from build123d import *

# Parameters (mm, degrees)
SKETCH1_R              = 50
BOSS_EXTRUDE2_DEPTH    = 2
SPLIT1_SURFACE_1_BACK  = 156.576
SPLIT1_SURFACE_1_DEPTH = 313.152
SPLIT1_SURFACE_2_BACK  = 156.576
SPLIT1_SURFACE_2_DEPTH = 313.152
BODY_DELETE1_DEPTH     = 2
BOSS_EXTRUDE3_DEPTH    = 2
BOSS_EXTRUDE5_START    = -2
SKETCH4_W              = 2
SKETCH4_H              = 5
BOSS_EXTRUDE5_DEPTH    = 2


# Read off the part's stored shape, not the designer's step: Body-Delete1
with BuildPart() as part:
    # Sketch1 → Boss-Extrude2 (new body)
    with BuildSketch(Plane(origin=(0, 0, 0), x_dir=(1, 0, 0), z_dir=(0, 1, 0))):
        with BuildLine():
            Line((22.912878475, 50), (30, 50))
            Line((30, 50), (30, 55))
            Line((30, 55), (0, 55))
            ThreePointArc((0, 55), (-11.7260394, -53.735463151), (22.912878475, 50))
        make_face()
        with Locations(Location((0, 0, 0), (0, 0, 270))):
            Circle(SKETCH1_R, mode=Mode.SUBTRACT)
    extrude(amount=BOSS_EXTRUDE2_DEPTH)


with BuildPart() as body_2:
    # Split1: the piece behind the surface
    add(part.part)
    # Split1 surface: a surface, the sketch's curves swept straight by 313.152 mm
    with BuildLine(Plane(origin=(0, 2, 0), x_dir=(1, 0, 0), z_dir=(0, 1, 0)).offset(-SPLIT1_SURFACE_1_BACK), mode=Mode.PRIVATE) as split1_surface_1_path:
        Line((0, 50), (71.831983425, 50))
        Line((71.831983425, 50), (71.831983425, -59.181674134))
        Line((71.831983425, -59.181674134), (-65.509549092, -59.181674134))
        Line((-65.509549092, -59.181674134), (-65.509549092, 0))
        Line((-65.509549092, 0), (0, 0))
        Line((0, 0), (0, 50))
    split1_surface_1 = Shell.extrude(split1_surface_1_path.wire(), (0 * SPLIT1_SURFACE_1_DEPTH, 1 * SPLIT1_SURFACE_1_DEPTH, 0 * SPLIT1_SURFACE_1_DEPTH))
    split(bisect_by=split1_surface_1, keep=Keep.BOTTOM)

    # Body-Delete1 outline → Body-Delete1 (cut)
    with BuildSketch(Plane(origin=(0, 0, 0), x_dir=(1, 0, 0), z_dir=(0, 1, 0))):
        with BuildLine():
            ThreePointArc((-55, 0), (29.705148408, -46.28827236), (22.912878475, 50))
            Line((22.912878475, 50), (0, 50))
            ThreePointArc((0, 50), (35.355339059, -35.355339059), (-50, 0))
            Line((-50, 0), (-55, 0))
        make_face()
    extrude(amount=BODY_DELETE1_DEPTH, mode=Mode.SUBTRACT)


with BuildPart() as part_1:
    add(part.part)

    # Split1: split by a surface, the side it looks to stays
    # Split1 surface: a surface, the sketch's curves swept straight by 313.152 mm
    with BuildLine(Plane(origin=(0, 2, 0), x_dir=(1, 0, 0), z_dir=(0, 1, 0)).offset(-SPLIT1_SURFACE_2_BACK), mode=Mode.PRIVATE) as split1_surface_2_path:
        Line((0, 50), (71.831983425, 50))
        Line((71.831983425, 50), (71.831983425, -59.181674134))
        Line((71.831983425, -59.181674134), (-65.509549092, -59.181674134))
        Line((-65.509549092, -59.181674134), (-65.509549092, 0))
        Line((-65.509549092, 0), (0, 0))
        Line((0, 0), (0, 50))
    split1_surface_2 = Shell.extrude(split1_surface_2_path.wire(), (0 * SPLIT1_SURFACE_2_DEPTH, 1 * SPLIT1_SURFACE_2_DEPTH, 0 * SPLIT1_SURFACE_2_DEPTH))
    split(bisect_by=split1_surface_2, keep=Keep.TOP)

    # Sketch3 → Boss-Extrude3 (add)
    with BuildSketch(Plane(origin=(0, 2, 0), x_dir=(1, 0, 0), z_dir=(0, 1, 0))):
        Polygon((30, 50), (30, 48), (25, 48), (25, 52), (30, 52), align=None)
        Polygon((22, 50), (22, 48), (17, 48), (17, 52), (22, 52), align=None)
    extrude(amount=-BOSS_EXTRUDE3_DEPTH)

    # Sketch4 → Boss-Extrude5 (add)
    with BuildSketch(Plane(origin=(0, 2, 0), x_dir=(1, 0, 0), z_dir=(0, 1, 0)).offset(BOSS_EXTRUDE5_START)):
        with Locations((-47, 2.5)):
            Rectangle(SKETCH4_W, SKETCH4_H)
        with BuildLine():
            ThreePointArc((-48, 14), (-49.497474683, 7.071067812), (-50, 0))
            Line((-50, 0), (-48, 0))
            Line((-48, 0), (-48, 5))
            Line((-48, 5), (-48, 14))
        make_face()
    extrude(amount=BOSS_EXTRUDE5_DEPTH)


solid = part_1.part
CAD build for the part. Positions are in the model's coordinates, mm. A direction names the side the tool comes from. Give positions to 0.01 mm unless a question says otherwise; leave off trailing zeros. Write each loop counter-clockwise with the first axis right and the second up, starting at its lowest first coordinate (ties: lowest second). Pieces come first, ordered by that corner, then holes. Notation, with made-up numbers: (71.25, 16) - (129.25, 16) arc R26 cw to (129.25, 41) - close; hole circle Ø11 at (3.25, -19.75). An arc over 180 degrees is marked (long way). Answer as CSV lines item,"result".
Q1. Flat gauge pins, fed straight in: pin 1 Ø0.6 at (x, y) = (24, 1) entering from +Z; pin 2 Ø0.6 at (x, y) = (27.5, 1) entering from +Z; pin 3 Ø0.6 at (y, z) = (0.5, -7.5) entering from +X. Where does each tip first touch, or does it go through?
Result set:
pin 1,"z = -50"
pin 2,"z = -48"
pin 3,"x = -48"
Q2. Band-saw the part on A-A (y = 0.65). Give the cut face in (x, z), and give its area (3 significant figures).
Result set:
outline,"(-55, 0) arc R55 ccw to (0, -55) - (30, -55) - (30, -48) - (25, -48) - (25, -50) - (22, -50) - (22, -48) - (17, -48) - (17, -50) - (0, -50) arc R50 cw to (-48, -14) - (-48, -5) - (-46, -5) - (-46, 0) - close"
area,"611 mm²"
Q3. Band-saw the part on C-C (z = -11). Give the cut face in (x, y), and give its area (3 significant figures).
Result set:
outline,"(-53.89, 0) - (-48, 0) - (-48, 2) - (-53.89, 2) - close"
area,"11.8 mm²"
Q4. Band-saw the part on B-B (x = 20.5). Give the cut face in (y, z), and give its area (3 significant figures).
Result set:
outline,"(0, -55) - (2, -55) - (2, -48) - (0, -48) - close"
area,"14.0 mm²"
Q5. Pull direction X, two halves, no side cores. Call faces 1 (the face through (-25, 2, -44)), 2 (the face through (30, 1, -51)), 3 (the face through (8, 1, -50)): released by +X, released by -X, zero draft, split by the parting line, or undercut.
Result set:
face 1,"zero draft"
face 2,"released by +X"
face 3,"undercut"
Q6. Drill centre lines: line 1 (Z direction, x = 12, y = 1.5); line 2 (X direction, y = 1.5, z = -29.5); line 3 (Z direction, x = -40, y = 0.45). Where is each one in solid material? Low to high. Write a range as from..to.
Result set:
line 1,"-55..-50"
line 2,"-46.42..-40.37"
line 3,"-37.75..-30"
Q7. 3-axis set-ups, long thin cutter, end or side, ignore diameter. For faces 4 (the face through (25, 1, -49)), 5 (the face through (-46, 1, -2)), 6 (the face through (-38.461, 0.986, -39.316)), 7 (the face through (15, 1, -55)), 8 (the face through (-48, 1, -9)): which of +Z, -Z, +X, -X, +Y, -Y reach the whole face in a straight line?
Result set:
face 4,"+Z, +Y, -Y"
face 5,"+Z, +X, +Y, -Y"
face 6,"-Z, -X, +Y, -Y"
face 7,"-Z, +X, -X, +Y, -Y"
face 8,"+X, +Y, -Y"
